Read the model definition and answer for the solid it produces. Units are mm, in the model's axes. Coordinates: 2 decimals unless noted, no trailing zeros. Order: outer loops, then holes, each group sorted by start corner. A loop starts at its lowest first (then second) coordinate and runs counter-clockwise, first axis right, second up. Notation, with made-up numbers: M -7.5,11 L 9.5,11 A37 ccw 9.5,49 Z; hole C 1,1.25 d2. An arc over 180 degrees is marked long. Put each result on its own line as item: value.
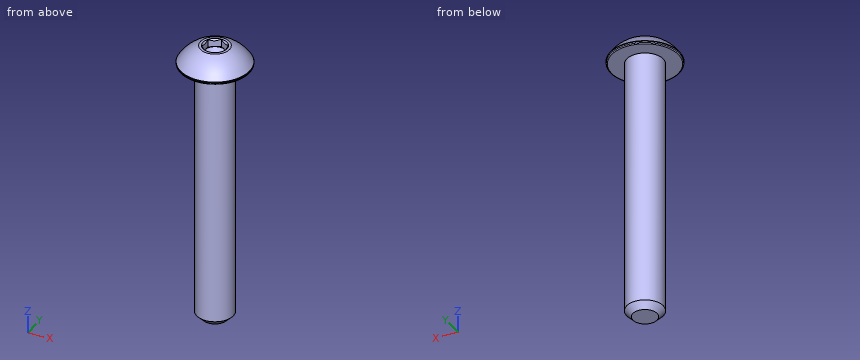
from build123d import *

# Parameters (mm, degrees)
CUT_EXTRUDE1_START = 12.88542
CUT_EXTRUDE1_DEPTH = 1.74168
SKETCH4_R          = 1.14567944
CUT_EXTRUDE2_DEPTH = 0.74168
CUT_EXTRUDE2_DRAFT = -45
FILLET1_R          = 0.09271


with BuildPart() as part:
    # Sketch2 → Revolve1 (revolve)
    with BuildSketch(Plane(origin=(0, 0, 0), x_dir=(0, 0, -1), z_dir=(1, 0, 0))):
        with BuildLine():
            Line((-13.6271, 0.9921875), (-13.6271, 1.3890625))
            ThreePointArc((-13.6271, 1.3890625), (-12.975897643, 2.494669105), (-11.999685714, 3.3274))
            Line((-11.999685714, 3.3274), (-11.7729, 3.28741156))
            Line((-11.7729, 3.28741156), (-11.7729, 1.7526))
            Line((-11.7729, 1.7526), (13.0317875, 1.7526))
            Line((13.0317875, 1.7526), (13.6271, 1.1572875))
            Line((13.6271, 1.1572875), (13.6271, 0))
            Line((13.6271, 0), (-12.31258028, 0))
            Line((-12.31258028, 0), (-12.88542, 0.9921875))
            Line((-12.88542, 0.9921875), (-13.6271, 0.9921875))
        make_face()
    revolve(axis=Axis((0, 0, 13.6271), (0, 0, -1)))

    # Sketch3 → Cut-Extrude1 (cut, through all)
    with BuildSketch(Plane.XY.offset(CUT_EXTRUDE1_START)):
        Polygon((0, 1.14567944), (-0.9921875, 0.57283972), (-0.9921875, -0.57283972), (0, -1.14567944), (0.9921875, -0.57283972), (0.9921875, 0.57283972), align=None)
    extrude(amount=CUT_EXTRUDE1_DEPTH, mode=Mode.SUBTRACT)


with BuildPart() as cut_extrude2_tool:
    # Sketch4 → Cut-Extrude2 (with draft: the straight prism first)
    with BuildSketch(Plane.XY.offset(13.6271)):
        Circle(SKETCH4_R)
    extrude(amount=-CUT_EXTRUDE2_DEPTH)
    # Cut-Extrude2: the draft: its side faces are tilted about the plane it starts from
    cut_extrude2_sides = [cut_extrude2_tool.faces().sort_by_distance(p)[0] for p in [
        (-1.14567944, 0, 13.25626),
    ]]
    draft(cut_extrude2_sides, Plane.XY.offset(13.6271), CUT_EXTRUDE2_DRAFT)


with BuildPart() as part_1:
    add(part.part)

    # Cut-Extrude2: cut by cut_extrude2_tool
    add(cut_extrude2_tool.part, mode=Mode.SUBTRACT)

    # Fillet1
    fillet1_edges = [part_1.edges().sort_by_distance(p)[0] for p in [
        (0, -3.28741156, 11.7729),
        (0, -3.3274, 11.999685714),
    ]]
    fillet(fillet1_edges, radius=FILLET1_R)


solid = part_1.part
Q1. Consider line 1 along Z through (x, y) = (0, -1); line 2 along Y through (x, z) = (0.5, 3.25); line 3 along Z through (x, y) = (-1.25, 2). Determine where each line is inside the solid, lowest interval first.
Answers below:
line 1: z = -13.63 to 12.89
line 2: y = -1.68 to 1.68
line 3: z = 11.77 to 13.09
Q2. Find section A-A on z = -11.75. Write down the section's boundary in (x, y), plus the area to 3 significant figures.
Answers below:
outline: C 0,0 d3.51
area: 9.65 mm^2
Q3. Given pin 1 (2 mm diameter, centred on x = -0.5, y = -1.5, fed in from +Z); pin 2 (1 mm diameter, centred on y = 0, z = -3, fed in from -X); pin 3 (3 mm diameter, centred on x = -1.5, z = 5, fed in from +Y), each flat-ended and moving along its own axis, determine where each tip first touches the part or whether it passes through.
Answers below:
pin 1: stops at z = 13.63
pin 2: stops at x = -1.75
pin 3: stops at y = 1.75
